The listing builds one solid part. Answer for the finished solid, in the listing's coordinates (mm). Give positions to 0.01 mm unless a question says otherwise; leave off trailing zeros. Write each loop counter-clockwise with the first axis right and the second up, starting at its lowest first coordinate (ties: lowest second). Pieces come first, ordered by that corner, then holes. Notation, with made-up numbers: (50, 48.5) -> (69, 48.5) arc R15 cw to (69, 57.5) -> close; hole circle Ø5 at (10.25, 28). An arc over 180 degrees is marked (long way). Use CSV: the item, a comma, the result in double quotes. Start each with the question number.
from build123d import *

# Parameters (mm, degrees)
SKETCH1_R           = 17
SKETCH1_R_2         = 8.5
BOSS_EXTRUDE1_DEPTH = 1
CUT_EXTRUDE1_START  = -2
SKETCH2_R           = 1.5
CUT_EXTRUDE1_DEPTH  = 3
CIRPATTERN1_COUNT   = 8


with BuildPart() as part:
    # Sketch1 → Boss-Extrude1 (new body)
    with BuildSketch(Plane.XY):
        Circle(SKETCH1_R)
        Circle(SKETCH1_R_2, mode=Mode.SUBTRACT)
    extrude(amount=BOSS_EXTRUDE1_DEPTH)

    # Sketch2 → Cut-Extrude1 (cut)
    with BuildSketch(Plane.XY.offset(1).offset(CUT_EXTRUDE1_START)):
        with Locations((0, 12)):
            Circle(SKETCH2_R)
    cut_extrude1 = extrude(amount=CUT_EXTRUDE1_DEPTH, mode=Mode.SUBTRACT)

    # CirPattern1: Cut-Extrude1 ×8 about axis
    cirpattern1_axis = Axis((0, 0, 0), (0, 0, 1))
    for i in range(1, CIRPATTERN1_COUNT):
        add(cut_extrude1.rotate(cirpattern1_axis, i * 360 / CIRPATTERN1_COUNT), mode=Mode.SUBTRACT)


solid = part.part
Q1. Straight lines are drawn through the part: L1, parallel to Y at x = 0, z = 0.35; L2, parallel to X at y = 1, z = 0.7; L3, parallel to Y at x = -13, z = 0.4. For each, find the intervals that lie inside material, in ascending order.
Q2. Section C-C on y = 4.5 is taken. Give the vertices of the cut face in (x, z), then the cut area to 3 significant figures.
Q3. Section D-D on z = 0.8 is taken. State how many separate pieces and enclosed holes the cut face has, then the cut area to 3 significant figures.
Q4. The mould has two halves that part along X. Classify faces 1 (the face through (8.7, -7, 0.5)), 2 (the face through (-8, -4, 1)), 3 (the face through (9.139, 14.334, 0.493)), 4 (the face through (-9.59, 7.47, 0.49)): +X half, -X half, draft (parallel to the pull), parting line (faces both ways), or undercut.
Q5. Section A-A on y = 0 is taken. Give the vertices of the cut face in (x, z), then the cut area to 3 significant figures.
Output:
1,L1,"-17 to -13.5, -10.5 to -8.5, 8.5 to 10.5, 13.5 to 17"
1,L2,"-16.97 to -13.12, -10.88 to -8.44, 8.44 to 10.88, 13.12 to 16.97"
1,L3,"-10.95 to -1.12, 1.12 to 10.95"
2,outline,"(-16.39, 0) -> (-7.21, 0) -> (-7.21, 1) -> (-16.39, 1) -> close; (7.21, 0) -> (16.39, 0) -> (16.39, 1) -> (7.21, 1) -> close"
2,area,"18.4 mm²"
3,separate pieces,"1"
3,enclosed holes,"9"
3,area,"624 mm²"
4,face 1,"undercut"
4,face 2,"draft"
4,face 3,"parting line"
4,face 4,"undercut"
5,outline,"(-17, 0) -> (-13.5, 0) -> (-13.5, 1) -> (-17, 1) -> close; (-10.5, 0) -> (-8.5, 0) -> (-8.5, 1) -> (-10.5, 1) -> close; (8.5, 0) -> (10.5, 0) -> (10.5, 1) -> (8.5, 1) -> close; (13.5, 0) -> (17, 0) -> (17, 1) -> (13.5, 1) -> close"
5,area,"11.0 mm²"
